Build history of the part. All positions in model axes, mm. A direction names the side the tool comes from. Give positions to 0.01 mm unless a question says otherwise; leave off trailing zeros. Write each loop counter-clockwise with the first axis right and the second up, starting at its lowest first coordinate (ties: lowest second). Pieces come first, ordered by that corner, then holes. Notation, with made-up numbers: M 66,-1.75 L 87,-1.75 A22 ccw 87,19.25 Z; hole C 9.25,-4.75 d8. An arc over 180 degrees is marked long. Return JSON: item names as keys, results as strings. Group by question number.
Q1. Band-saw the part on C-C, the plane x = -20. Give the cut face in (y, z).
Q2. Band-saw the part on D-D, the plane y = 15.1. Give the cut face in (x, z), then the cut area to 3 significant figures.
Q3. Band-saw the part on B-B, the plane y = 25. Give the cut face in (x, z).
Q4. Flat gauge pins, fed straight in: pin 1 Ø3 at (x, z) = (-72, 10.5) entering from +Y; pin 2 Ø3 at (y, z) = (72, -11) entering from -X; pin 3 Ø15.5 at (x, z) = (-21, 6) entering from +Y. Where does each tip first touch, or does it go through?
Q5. Pull direction Z, two halves, no side cores. Call faces 1 (the cylindrical face through (-4.056, 54.423, -11.778)), 2 (the cylindrical face through (-15.1, 13, 0.4)), 3 (the flat face through (-19, 16, 29)): +Z half, -Z half, draft (parallel to the pull), parting line (faces both ways), or undercut.
Q6. Wall check: probe 1 along Z at (x, y) = (-6.5, 54); probe 2 along X at (y, z) = (6, 15); probe 3 along X at (y, z) = (50, 13). Give the ranges that are in metal, low to high.
Q7. Tool access for faces 4 (the flat face through (-40, 0, 0)), 5 (the flat face through (-47, 8, 0)), 6 (the flat face through (-19, 4.5, 0)): list every direction of +Z, -Z, +X, -X, +Y, -Y with a clear straight run to the whole face (end or side of a thin tool).
Q8. Band-saw the part on A-A, the plane z = -15. Count the separate pieces of the cut face and the enclosed holes in it, then the cut area to 3 significant figures.
from build123d import *

# Parameters (mm, degrees)
EXTRUDE_1_DEPTH     = 29
SKETCH_2_R          = 3.25
CUT_EXTRUDE_1_DEPTH = 9
SKETCH_3_R          = 3.25
CUT_EXTRUDE_2_DEPTH = 9


with BuildPart() as part:
    # Эскиз1 → Бобышка-Вытянуть1 (new body, symmetric)
    with BuildSketch(Plane.XY):
        Polygon((-78, 0), (0, 0), (0, 78), (-8, 78), (-8, 68.5), (-7.5, 68), (-8, 67.5), (-8, 54.5), (-7.5, 54), (-8, 53.5), (-8, 40.5), (-7.5, 40), (-8, 39.5), (-8, 30), (-30, 8), (-39.5, 8), (-40, 7.5), (-40.5, 8), (-53.5, 8), (-54, 7.5), (-54.5, 8), (-67.5, 8), (-68, 7.5), (-68.5, 8), (-78, 8), align=None)
        with BuildLine():
            Line((-4.5, 12), (-4.5, 26.136038969))
            ThreePointArc((-4.5, 26.136038969), (-5.117316568, 27.059918502), (-6.207106781, 26.843145751))
            Line((-6.207106781, 26.843145751), (-26.843145751, 6.207106781))
            ThreePointArc((-26.843145751, 6.207106781), (-27.059918502, 5.117316568), (-26.136038969, 4.5))
            Line((-26.136038969, 4.5), (-12, 4.5))
            Line((-12, 4.5), (-12, 7.9))
            ThreePointArc((-12, 7.9), (-14.899137803, 9.100862197), (-16.1, 12))
            ThreePointArc((-16.1, 12), (-15.1, 13), (-14.1, 12))
            ThreePointArc((-14.1, 12), (-10.51507576, 10.51507576), (-12, 14.1))
            ThreePointArc((-12, 14.1), (-13, 15.1), (-12, 16.1))
            ThreePointArc((-12, 16.1), (-9.100862197, 14.899137803), (-7.9, 12))
            Line((-7.9, 12), (-4.5, 12))
        make_face(mode=Mode.SUBTRACT)
    extrude(amount=EXTRUDE_1_DEPTH, both=True)

    # Эскиз2 → Вырез-Вытянуть1 (cut, through all)
    with BuildSketch(Plane.ZY.offset(8)):
        with Locations(Location((-15, 54, 0), (0, 0, 270))):  # turned: the seam where the file's is
            Circle(SKETCH_2_R)
        with Locations(Location((15, 54, 0), (0, 0, 270))):  # turned: the seam where the file's is
            Circle(SKETCH_2_R)
    extrude(amount=-CUT_EXTRUDE_1_DEPTH, mode=Mode.SUBTRACT)

    # Эскиз3 → Вырез-Вытянуть2 (cut, through all)
    with BuildSketch(Plane(origin=(0, 8, 0), x_dir=(1, 0, 0), z_dir=(0, 1, 0))):
        with Locations(Location((-54, -15, 0), (0, 0, 180))):  # turned: the seam where the file's is
            Circle(SKETCH_3_R)
        with Locations(Location((-54, 15, 0), (0, 0, 180))):  # turned: the seam where the file's is
            Circle(SKETCH_3_R)
    extrude(amount=-CUT_EXTRUDE_2_DEPTH, mode=Mode.SUBTRACT)


solid = part.part
From the geometry:
{
 "1": {"outline": "M 0,-29 L 4.5,-29 L 4.5,29 L 0,29 Z; M 13.05,-29 L 18,-29 L 18,29 L 13.05,29 Z"},
 "2": {"outline": "M -22.9,-29 L -17.95,-29 L -17.95,29 L -22.9,29 Z; M -13,-29 L -9.32,-29 L -9.32,29 L -13,29 Z; M -4.5,-29 L 0,-29 L 0,29 L -4.5,29 Z", "area": "762 mm^2"},
 "3": {"outline": "M -13,-29 L -8.05,-29 L -8.05,29 L -13,29 Z; M -4.5,-29 L 0,-29 L 0,29 L -4.5,29 Z"},
 "4": {"pin 1": "stops at y = 8", "pin 2": "stops at x = -8", "pin 3": "stops at y = 24.75"},
 "5": {"face 1": "undercut", "face 2": "draft", "face 3": "+Z half"},
 "6": {"probe 1": "z = -29 to -18.25, -11.75 to 11.75, 18.25 to 29", "probe 2": "x = -78 to -57.25, -50.75 to -27, -12 to 0", "probe 3": "x = -8 to 0"},
 "7": {"face 4": "+Z, -Z, +X, -X, -Y", "face 5": "+Z, -Z, -X, +Y", "face 6": "+Z, -Z"},
 "8": {"separate pieces": "3", "enclosed holes": "1", "area": "1,110 mm^2"}
}
